```python
from build123d import *

# Parameters (mm, degrees)
SKETCH4_R          = 5
CUT_EXTRUDE1_DEPTH = 8
SKETCH5_R          = 3
CUT_EXTRUDE2_DEPTH = 48
SKETCH6_R          = 1
CUT_EXTRUDE3_DEPTH = 48


with BuildPart() as part:
    # Sketch2 → Revolve1 (revolve)
    with BuildSketch(Plane.XY, mode=Mode.PRIVATE) as revolve1_sk:
        Polygon((0, 0), (25, 0), (25, 3.419684485), (25, 48), (15.707106781, 48), (15, 47.292893219), (15, 28), (0, 28), align=None)
    revolve(revolve1_sk.sketch.rotate(Axis((0, 0, 0), (0, 1, 0)), 90), axis=Axis((0, 0, 0), (0, 1, 0)))

    # Sketch4 → Cut-Extrude1 (cut)
    with BuildSketch(Plane(origin=(0, 28, 0), x_dir=(1, 0, 0), z_dir=(0, 1, 0))):
        with Locations(Location((0, 0, 0), (0, 0, 270))):
            Circle(SKETCH4_R)
    extrude(amount=-CUT_EXTRUDE1_DEPTH, mode=Mode.SUBTRACT)

    # Sketch5 → Cut-Extrude2 (cut)
    with BuildSketch(Plane(origin=(0, 20, 0), x_dir=(1, 0, 0), z_dir=(0, 1, 0))):
        with Locations(Location((0, 0, 0), (0, 0, 270))):
            Circle(SKETCH5_R)
    extrude(amount=-CUT_EXTRUDE2_DEPTH, mode=Mode.SUBTRACT)

    # Sketch6 → Cut-Extrude3 (cut)
    with BuildSketch(Plane.XY):
        with Locations((0, 24)):
            Circle(SKETCH6_R)
    extrude(amount=-CUT_EXTRUDE3_DEPTH, mode=Mode.SUBTRACT)


solid = part.part
```
The model under review builds one solid part; all positions refer to its coordinate system, in mm. A direction names the side the tool comes from. Coordinates: 2 decimals unless noted, no trailing zeros. Order: outer loops, then holes, each group sorted by start corner. A loop starts at its lowest first (then second) coordinate and runs counter-clockwise, first axis right, second up. Notation, with made-up numbers: M -28.5,-25.5 L 2.5,-25.5 A13 ccw 2.5,-10.5 Z; hole C 0,28 d8. An arc over 180 degrees is marked long. One line per question, with ' | ' between items.
(1) The part is to be moulded in two halves that separate along X. For faces 1 (the face through (-7.509, 24.336, -23.846)), 2 (the face through (-4, 28, 4)), 3 (the face through (-3.3, 20, -0.1)), 4 (the face through (5, 0, 0)), say which applies: +X half, -X half, draft (parallel to the pull), parting line (faces both ways), or undercut.
Geometry results:
face 1: parting line | face 2: undercut | face 3: undercut | face 4: draft
(2) Insertion check: pin 1 (11 mm diameter, centred on x = -1, z = 2, fed in from +Y); pin 2 (12 mm diameter, centred on x = -7, y = 14, fed in from +Z); pin 3 (1.5 mm diameter, centred on x = -2.5, y = 37.5, fed in from +Z). Each pin has a flat end and moves straight along its axis. Give the tip position at first contact, or say it passes through.
Geometry results:
pin 1: stops at y = 28 | pin 2: stops at z = 24.98 | pin 3: stops at z = 24.94
(3) Machinability: for faces 5 (the face through (0, 23, -15)), 6 (the face through (0.9, 10.14, 2.86)), 7 (the face through (1.5, 24.06, 4.77)), which of the approach directions +Z, -Z, +X, -X, +Y, -Y give a long, thin tool a straight path to every point of the face, cutting with its end or side? Answer none if there is none.
Geometry results:
face 5: -Z | face 6: +Y, -Y | face 7: +Y
(4) For probe 1 along X at (y, z) = (14.25, 0); probe 2 along Y at (x, z) = (14, -3); probe 3 along X at (y, z) = (35, 0), list the stretches that pass through material, from the lowest coordinate up. Write a range as from..to.
Geometry results:
probe 1: x = -25..-3, 3..25 | probe 2: y = 0..28 | probe 3: x = -25..-15, 15..25
(5) Add section D-D, the plane z = -20.5. Write out the cut boundary in (x, y).
Geometry results:
outline: M -14.31,0 L 14.31,0 L 14.31,48 L -14.31,48 Z; hole C 0,24 d2
(6) Add section B-B, the plane y = 43. Write out the cut boundary in (x, z).
Geometry results:
outline: C 0,0 d50; hole C 0,0 d30
(7) Add section C-C, the plane y = 24. Write out the cut boundary in (x, z).
Geometry results:
outline: M -1,-24.98 L -1,-4.9 A5 cw long 1,-4.9 L 1,-24.98 A25 ccw long Z
(8) Add section A-A, the plane x = 0. Write out the cut boundary in (y, z), then the cut area to 3 significant figures.
Geometry results:
outline: M 0,-25 L 23,-25 L 23,-5 L 20,-5 L 20,-3 L 0,-3 Z; M 0,3 L 20,3 L 20,5 L 28,5 L 28,15 L 47.29,15 L 48,15.71 L 48,25 L 0,25 Z; M 25,-25 L 48,-25 L 48,-15.71 L 47.29,-15 L 28,-15 L 28,-5 L 25,-5 Z | area: 1,560 mm²
